Check sheet for the modelled part. Datum: model origin and axes. Units: mm. Face numbers are marked on the shaded views. A direction names the side the tool comes from. Coordinates: 2 decimals unless noted, no trailing zeros. Loops run counter-clockwise (first coordinate to the right, second up) from the corner with the lowest first, then second, coordinate; pieces in that order, holes last. Notation, with made-up numbers: (-24, 38) -> (-13, 38) arc R29 cw to (-13, 73) -> close; hole circle Ø7 at (17, -36). An arc over 180 degrees is marked (long way). Use CSV: the item, a comma, the result in double quotes.
```python
from build123d import *

# Parameters (mm, degrees)
BOSS_EXTRUDE1_DEPTH = 1.27
BOSS_EXTRUDE3_DEPTH = 17.78
SKETCH5_W           = 38.1
SKETCH5_H           = 19.05
BOSS_EXTRUDE4_DEPTH = 2.54
FILLET1_R           = 7.62
CUT_EXTRUDE5_REACH  = 40.1
FILLET3_R           = 2.54


with BuildPart() as part:
    # Sketch1 → Boss-Extrude1 (new body)
    with BuildSketch(Plane(origin=(0, 0, 0), x_dir=(1, 0, 0), z_dir=(0, 1, 0))):
        with BuildLine():
            Line((0, 0), (38.1, 0))
            Line((38.1, 0), (38.1, -25.4))
            ThreePointArc((38.1, -25.4), (19.05, -44.45), (0, -25.4))
            Line((0, -25.4), (0, 0))
        make_face()
    extrude(amount=BOSS_EXTRUDE1_DEPTH)

    # Sketch3 → Boss-Extrude3 (add)
    with BuildSketch(Plane(origin=(0, 1.27, 0), x_dir=(1, 0, 0), z_dir=(0, 1, 0))):
        with BuildLine():
            Line((0, 0), (0, -25.4))
            ThreePointArc((0, -25.4), (19.05, -44.45), (38.1, -25.4))
            Line((38.1, -25.4), (38.1, 0))
            Line((38.1, 0), (36.83, 0))
            Line((36.83, 0), (36.83, -25.4))
            ThreePointArc((36.83, -25.4), (19.05, -43.18), (1.27, -25.4))
            Line((1.27, -25.4), (1.27, 0))
            Line((1.27, 0), (0, 0))
        make_face()
    extrude(amount=BOSS_EXTRUDE3_DEPTH)

    # Sketch5 → Boss-Extrude4 (add)
    with BuildSketch(Plane(origin=(0, 0, 0), x_dir=(-1, 0, 0), z_dir=(0, 0, -1))):
        with Locations((-19.05, 9.525)):
            Rectangle(SKETCH5_W, SKETCH5_H)
    extrude(amount=BOSS_EXTRUDE4_DEPTH)

    # Fillet1
    fillet1_edges = [part.edges().sort_by_distance(p)[0] for p in [
        (19.05, 1.27, 0),
        (36.83, 1.27, 12.7),
        (19.05, 1.27, 43.18),
        (1.27, 1.27, 12.7),
    ]]
    fillet(fillet1_edges, radius=FILLET1_R)

    # Sketch9 → Cut-Extrude5 (cut, up to next)
    with BuildSketch(Plane.ZY, mode=Mode.PRIVATE) as cut_extrude5_sk1:
        with BuildLine():
            Line((24.13, 35.56), (26.67, 35.56))
            ThreePointArc((26.67, 35.56), (43.18, 19.05), (26.67, 2.54))
            Line((26.67, 2.54), (24.13, 2.54))
            ThreePointArc((24.13, 2.54), (7.62, 19.05), (24.13, 35.56))
        make_face()
    cut_extrude5_tool1 = extrude(cut_extrude5_sk1.sketch, amount=-CUT_EXTRUDE5_REACH, mode=Mode.PRIVATE) & part.part
    add(cut_extrude5_tool1.solids().sort_by_distance((0, 19.05, 25.4))[0], mode=Mode.SUBTRACT)

    # Fillet3
    fillet3_edges = [part.edges().sort_by_distance(p)[0] for p in [
        (0.635, 19.05, 7.62),
    ]]
    fillet(fillet3_edges, radius=FILLET3_R)


solid = part.part
```
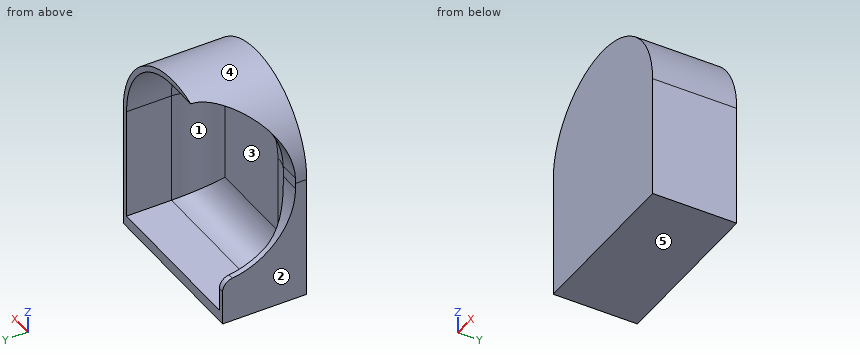
1) Draft check along X on the marked faces 3, 4 and 5. Enter one of: released by +X, released by -X, zero draft, split by the parting line, or undercut.
Answer below:
face 3,"undercut"
face 4,"split by the parting line"
face 5,"zero draft"
2) Thickness scan on line 1 along X through (y, z) = (14.75, 3); line 2 along Z through (x, y) = (19, 8.5); line 3 along Y through (x, z) = (21, 16.5). Record the ranges inside material, lowest first. Write a range as from..to.
Answer below:
line 1,"x = 0..1.27, 36.83..38.1"
line 2,"z = -2.54..0.01, 43.17..44.45"
line 3,"y = 0..1.27"
3) Access from +Z, -Z, +X, -X, +Y, -Y to the whole of each face (thin tool, end or side, straight path). Record for the marked faces 1 and 2.
Answer below:
face 1,"+Y"
face 2,"+Z, -Z, -X, +Y, -Y"
4) Cross-section at A-A on y = 11.25. Record the boundary of the cut face in (x, z).
Answer below:
outline,"(0, -2.54) -> (38.1, -2.54) -> (38.1, 25.4) arc R19.05 ccw to (8.44, 41.22) -> (10.94, 41.22) arc R17.78 cw to (36.83, 25.4) -> (36.83, 0) -> (1.27, 0) -> (1.27, 9.58) -> (0, 9.58) -> close"
5) Go/stop test with flat-tipped pins: pin 1 Ø3 at (x, y) = (10.5, 2.5) entering from +Z; pin 2 Ø1.5 at (y, z) = (12.5, 38.5) entering from -X; pin 3 Ø3 at (y, z) = (16.5, 15.5) entering from -X. Record where each tip stops, or that it passes through.
Answer below:
pin 1,"stops at z = 43.1"
pin 2,"stops at x = 30.2"
pin 3,"stops at x = 36.83"
6) Cross-section at B-B on y = 15.75. Record the boundary of the cut face in (x, z).
Answer below:
outline,"(0, -2.54) -> (38.1, -2.54) -> (38.1, 25.4) arc R19.05 ccw to (11.4, 42.85) -> (15.62, 42.85) arc R17.78 cw to (36.83, 25.4) -> (36.83, 0) -> (1.27, 0) -> (1.27, 7.95) -> (0, 7.95) -> close"
